Autodesk Inventor part; units mm, degrees
ref_plane "YZ Plane" through (0, 0, 0) normal (1, 0, 0) x (0, 1, 0)
ref_plane "XZ Plane" through (0, 0, 0) normal (0, 1, 0) x (-1, 0, 0)
ref_plane "XY Plane" through (0, 0, 0) normal (0, 0, 1) x (1, 0, 0)
sketch "Sketch1" plane through (0, 0, 0) normal (0, 0, 1) x (1, 0, 0)
  circle A0 centre (0, 0) radius 9
  circle A1 centre (0, 0) radius 7
  dimension "d0" = 18
  dimension "d1" = 2
extrude "Extrusion1" add sketch "Sketch1" along normal blind 120 contours A0 | A1
chamfer "Chamfer1" distance 0.2 angle 45 2 edges at (-9, 0, 0) (-9, 0, 120)
sketch "Sketch2" plane through (0, 0, 120) normal (0, 0, 1) x (1, 0, 0)
  circle A0 centre (0, 0) radius 9
hole "Hole1" at (0, 0, 120) direction (0, 0, -1) diameter 8.376 end through all
properties part number "buis 18 mm" material "Stainless Steel"
The listing builds one solid part. Answer for the finished solid, in the listing's coordinates (mm). Round coordinates to 2 decimals unless told otherwise and drop trailing zeros. Loops run counter-clockwise (first coordinate to the right, second up) from the corner with the lowest first, then second, coordinate; pieces in that order, holes last. Notation, with made-up numbers: M 77.5,58.25 L 112.5,58.25 A25 ccw 112.5,76.25 Z; hole C -16.5,17.5 d9. An arc over 180 degrees is marked long. Return JSON: item names as keys, results as strings.
Q1. Find section A-A, the plane x = 0. Determine the outline of the cut face in (y, z), plus the area to 3 significant figures.
Results list:
{"outline": "M -9,0.2 L -8.8,0 L -4.19,0 L -4.19,120 L -8.8,120 L -9,119.8 Z; M 4.19,0 L 8.8,0 L 9,0.2 L 9,119.8 L 8.8,120 L 4.19,120 Z", "area": "1,150 mm2"}
Q2. The mould has two halves that part along Y. Classify faces 1 (the face through (-1.172, -8.923, 59.163)), 2 (the face through (4, -2, 0)), 3 (the face through (-2.83, 3.087, 59.16)): released by +Y, released by -Y, zero draft, split by the parting line, or undercut.
Results list:
{"face 1": "split by the parting line", "face 2": "zero draft", "face 3": "undercut"}
Q3. Find section C-C, the plane z = 43. Determine the outline of the cut face in (x, y).
Results list:
{"outline": "C 0,0 d18; hole C 0,0 d8.38"}
Q4. Find the intervals of material crossed by line 1 along Y through (x, z) = (0, 93); line 2 along X through (y, z) = (-0.25, 70); line 3 along Y through (x, z) = (-3.25, 72), in increasing order. Write a range as from..to.
Results list:
{"line 1": "y = -9..-4.19, 4.19..9", "line 2": "x = -9..-4.18, 4.18..9", "line 3": "y = -8.39..-2.64, 2.64..8.39"}
Q5. Each of these flat-tipped pins is pushed along its axis until it touches: pin 1 Ø10 at (x, z) = (3.5, 25.5) entering from -Y; pin 2 Ø6.5 at (x, y) = (0, 0) entering from -Z; pin 3 Ø8 at (x, z) = (4.5, 70) entering from +Y; pin 4 Ø6 at (y, z) = (-6.5, 23) entering from -X. Where does it stop, or does it pass through?
Results list:
{"pin 1": "stops at y = -9", "pin 2": "passes through", "pin 3": "stops at y = 8.99", "pin 4": "stops at x = -8.29"}
